Geometry: final body of the model. Coordinates: model frame, mm. A direction names the side the tool comes from. Give positions to 0.01 mm unless a question says otherwise; leave off trailing zeros. Loops run counter-clockwise (first coordinate to the right, second up) from the corner with the lowest first, then second, coordinate; pieces in that order, holes last.
from build123d import *

# Parameters (mm, degrees)
SKETCH2_W               = 113.16294167
SKETCH2_H               = 44.385347151
CUT_EXTRUDE1_DEPTH      = 40.876559531
BOSS_EXTRUDE1_START     = -8
BOSS_EXTRUDE1_DEPTH     = 8
CORTAR_EXTRUIR1_DEPTH   = 3.5
SKETCH4_R               = 1.5
SALIENTE_EXTRUIR1_DEPTH = 2.5
CHAFL_N5_SIZE           = 0.5
SCALE1_SCALE            = 2.1714285


with BuildPart() as part:
    # Sketch1 → Revolve1 (revolve)
    with BuildSketch(Plane(origin=(0, 0, 0), x_dir=(1, 0, 0), z_dir=(0, 1, 0))):
        Polygon((21.5, 12.9), (16, 12.9), (16, 9.9), (12.5, 9.9), (12.5, 4.15), (17.55, 4.15), (17.55, -4.15), (12.5, -4.15), (12.5, -9.9), (16, -9.9), (16, -12.9), (21.5, -12.9), align=None)
    revolve(axis=Axis((0, 0, 0), (0, 0, -1)))

    # Sketch2 → Cut-Extrude1 (cut, through all)
    with BuildSketch(Plane(origin=(0, 0, -12.9), x_dir=(-1, 0, 0), z_dir=(0, 0, -1))):
        with Locations((0, -22.192673576)):
            Rectangle(SKETCH2_W, SKETCH2_H)
    extrude(amount=-CUT_EXTRUDE1_DEPTH, mode=Mode.SUBTRACT)

    # Sketch3 → Boss-Extrude1 (add)
    with BuildSketch(Plane.XY.offset(12.9).offset(BOSS_EXTRUDE1_START)):
        with BuildLine():
            ThreePointArc((9.901123545, 19.084489842), (15.202795796, 15.202795796), (19.084489842, 9.901123545))
            Line((19.084489842, 9.901123545), (22.894785555, 13.731141284))
            ThreePointArc((22.894785555, 13.731141284), (23.272346041, 23.272346041), (13.731141284, 22.894785555))
            Line((13.731141284, 22.894785555), (9.901123545, 19.084489842))
        make_face()
        with BuildLine():
            Line((-9.901123545, 19.084489842), (-13.731141284, 22.894785555))
            ThreePointArc((-13.731141284, 22.894785555), (-23.272346041, 23.272346041), (-22.894785555, 13.731141284))
            Line((-22.894785555, 13.731141284), (-19.084489842, 9.901123545))
            ThreePointArc((-19.084489842, 9.901123545), (-15.202795796, 15.202795796), (-9.901123545, 19.084489842))
        make_face()
    extrude(amount=BOSS_EXTRUDE1_DEPTH)

    # Croquis6 → Cortar-Extruir1 (cut)
    with BuildSketch(Plane.XY.offset(12.9)):
        Polygon((-15.331536888, 22.020767038), (-14.107322805, 17.45193788), (-17.45193788, 14.107322805), (-22.020767038, 15.331536888), (-23.244981122, 19.900366047), (-19.900366047, 23.244981122), align=None)
        Polygon((15.331536888, 22.020767038), (19.90036573, 23.244982303), (23.24497994, 19.900366363), (22.020767038, 15.331536888), (17.451938197, 14.107321624), (14.107323987, 17.451937564), align=None)
    extrude(amount=-CORTAR_EXTRUIR1_DEPTH, mode=Mode.SUBTRACT)

    # Sketch4 → Saliente-Extruir1 (add)
    with BuildSketch(Plane.XZ):
        with Locations(Location((-18.75, 8.525, 0), (0, 0, 90))):
            Circle(SKETCH4_R)
        with Locations(Location((18.75, -8.525, 0), (0, 0, 90))):
            Circle(SKETCH4_R)
        with Locations(Location((18.75, 8.525, 0), (0, 0, 90))):
            Circle(SKETCH4_R)
        with Locations(Location((-18.75, -8.525, 0), (0, 0, 90))):
            Circle(SKETCH4_R)
    extrude(amount=SALIENTE_EXTRUIR1_DEPTH)

    # Chaflán5
    chafl_n5_edges = [part.edges().sort_by_distance(p)[0] for p in [
        (-18.75, -2.5, 7.025),
        (18.75, -2.5, 7.025),
        (18.75, -2.5, -10.025),
        (-18.75, -2.5, -10.025),
    ]]
    chamfer(chafl_n5_edges, length=CHAFL_N5_SIZE)


with BuildPart() as part_1:
    # Scale1: scaled about (0, 12.592522151, 1.292940279)
    add(part.part.scale(SCALE1_SCALE).moved(Location((0, -14.751239335, -1.514587092))))


solid = part_1.part
Item 1: Section query A-A on z = 22.5. Return loops of the section in (x, y).
Values follow:
outline: (-49.71, 15.06) - (-41.44, 6.75) arc R46.69 ccw to (-46.69, -14.75) - (-34.74, -14.75) arc R34.74 cw to (34.74, -14.75) - (46.69, -14.75) arc R46.69 ccw to (41.44, 6.75) - (49.71, 15.06) arc R14.11 ccw (long way) to (29.82, 34.96) - (21.5, 26.69) arc R46.69 ccw to (-21.5, 26.69) - (-29.82, 34.96) arc R14.11 ccw (long way) to start; hole (-50.47, 28.46) - (-47.82, 18.54) - (-37.9, 15.88) - (-30.63, 23.14) - (-33.29, 33.07) - (-43.21, 35.72) - close; hole (30.63, 23.14) - (37.9, 15.88) - (47.82, 18.54) - (50.47, 28.46) - (43.21, 35.72) - (33.29, 33.07) - close
Item 2: Draft query along Z for faces 5 (the face through (-25.6, 30.77, 17.69)), 6 (the face through (37.485, -16.892, 16.573)), 7 (the face through (1, 24, 26.497)). Return one class per face: +Z half, -Z half, draft (parallel to the pull), parting line (faces both ways), or undercut.
Values follow:
face 5: draft
face 6: undercut
face 7: +Z half
Item 3: Section query C-C on x = 0. Return loops of the section in (y, z).
Values follow:
outline: (12.39, -23.01) - (19.99, -23.01) - (19.99, -29.53) - (31.93, -29.53) - (31.93, 26.5) - (19.99, 26.5) - (19.99, 19.98) - (12.39, 19.98) - (12.39, 7.5) - (23.36, 7.5) - (23.36, -10.53) - (12.39, -10.53) - close
Item 4: Pin query (flat end, axial travel): pin 1 (10 mm diameter, centred on x = -22, z = 19, fed in from +Y); pin 2 (6 mm diameter, centred on y = -9, z = -23.5, fed in from +X); pin 3 (10 mm diameter, centred on x = 41.5, z = 9, fed in from -Y); pin 4 (10 mm diameter, centred on x = -36, y = 30, fed in from +Z). Return the tip coordinate at first contact, or that it passes through.
Values follow:
pin 1: stops at y = 32.16
pin 2: stops at x = 46.6
pin 3: stops at y = -19.32
pin 4: stops at z = 26.5
Item 5: Set-up query: faces 1 (the face through (-37.535, -16.892, -20.732)), 2 (the face through (31.944, 28.035, 22.75)), 3 (the face through (-0.764, 19.983, -26.223)), 4 (the face through (-2, 13, 19.983)). Return all of +Z, -Z, +X, -X, +Y, -Y with unobstructed straight access to the full face (end or side cutting, diameter ignored); none if empty.
Values follow:
face 1: -Y
face 2: +Z
face 3: -Z, -Y
face 4: +Z, -Y
Item 6: Section query D-D on z = 12. Return loops of the section in (x, y), plus the area to 3 significant figures.
Values follow:
outline: (-49.71, 15.06) - (-41.44, 6.75) arc R46.69 ccw to (-46.69, -14.75) - (-27.14, -14.75) arc R27.14 cw to (27.14, -14.75) - (46.69, -14.75) arc R46.69 ccw to (41.44, 6.75) - (49.71, 15.06) arc R14.11 ccw (long way) to (29.82, 34.96) - (21.5, 26.69) arc R46.69 ccw to (-21.5, 26.69) - (-29.82, 34.96) arc R14.11 ccw (long way) to start
area: 3,530 mm2
Item 7: Ray query, probe 1 along Z at (x, y) = (-14, 13); probe 2 along X at (y, z) = (21, 21.5); probe 3 along X at (y, z) = (10.5, -24). Return the intervals inside material, ascending.
Values follow:
probe 1: z = -23.01 to -10.53, 7.5 to 19.98
probe 2: x = -53.83 to -48.48, -32.78 to 32.78, 48.48 to 53.83
probe 3: x = -39.27 to -23.86, 23.86 to 39.27
Item 8: Section query B-B on y = 0. Return loops of the section in (x, z).
Values follow:
outline: (-44.29, -29.53) - (-31.46, -29.53) - (-31.46, -23.01) - (-22.78, -23.01) - (-22.78, -10.53) - (-35.14, -10.53) - (-35.14, 7.5) - (-22.78, 7.5) - (-22.78, 19.98) - (-31.46, 19.98) - (-31.46, 26.5) - (-44.29, 26.5) - close; (22.78, -23.01) - (31.46, -23.01) - (31.46, -29.53) - (44.29, -29.53) - (44.29, 26.5) - (31.46, 26.5) - (31.46, 19.98) - (22.78, 19.98) - (22.78, 7.5) - (35.14, 7.5) - (35.14, -10.53) - (22.78, -10.53) - close
